The model under review builds one solid part; all positions refer to its coordinate system, in mm. Coordinates: 2 decimals unless noted, no trailing zeros. Write each loop counter-clockwise with the first axis right and the second up, starting at its lowest first coordinate (ties: lowest second). Pieces come first, ordered by that corner, then holes. Notation, with made-up numbers: (-9.5, -38.5) - (10.5, -38.5) arc R29 ccw to (10.5, -2.5) - close; hole circle Ø1 at (-27, 21). An arc over 180 degrees is marked (long way). Put each result on its own line as item: value.
Autodesk Inventor part; units mm, degrees
ref_plane "YZ Plane" through (0, 0, 0) normal (1, 0, 0) x (0, 1, 0)
ref_plane "XZ Plane" through (0, 0, 0) normal (0, 1, 0) x (-1, 0, 0)
ref_plane "XY Plane" through (0, 0, 0) normal (0, 0, 1) x (1, 0, 0)
sketch "Sketch3" plane through (0, 0, 0) normal (0, 1, 0) x (-1, 0, 0)
  line L0 (50, 50) -> (-50, 50)
  line L1 (-50, 50) -> (-50, -50)
  line L2 (-50, -50) -> (50, -50)
  line L3 (50, -50) -> (50, 50)
  line L4 (-50, -45) -> (50, -45) construction
  line L5 (-50, 45) -> (50, 45) construction
  line L6 (22.5, 50) -> (22.5, -50) construction
  line L7 (-22.5, 50) -> (-22.5, -50) construction
  circle A0 centre (-22.5, -45) radius 1.575
  circle A1 centre (-22.5, 45) radius 1.575
  circle A2 centre (22.5, 45) radius 1.575
  circle A3 centre (22.5, -45) radius 1.575
  point P0 (0, 0)
  dimension "d4" = 100
  dimension "d5" = 100
  dimension "d6" = 5
  dimension "d7" = 5
  dimension "d8" = 27.5
  dimension "d9" = 27.5
  dimension "d10" = 3.15
  dimension "d11" = 3.15
  dimension "d12" = 3.15
  dimension "d13" = 3.15
extrude "Extrusion1" add sketch "Sketch3" along normal blind 1
properties part number "CompCellScopeArray"
1. Consider section A-A on z = 45. State the section outline as (x, y) points (3 decimals).
Determined:
outline: (-50, 0) - (-24.075, 0) - (-24.075, 1) - (-50, 1) - close; (-20.925, 0) - (20.925, 0) - (20.925, 1) - (-20.925, 1) - close; (24.075, 0) - (50, 0) - (50, 1) - (24.075, 1) - close
2. To check wall thickness, follow probe 1 along Z at (x, y) = (-22.5, 0.5) (3 decimals). State the ranges of the line that lie inside material, in increasing order.
Determined:
probe 1: z = -50 to -46.575, -43.425 to 43.425, 46.575 to 50
3. The part is to be moulded in two halves that separate along X. For faces 1 (the cylindrical face through (23.661, 0.493, 43.936)), 2 (the flat face through (1, 0, 1)), say which applies: +X half, -X half, draft (parallel to the pull), parting line (faces both ways), or undercut.
Determined:
face 1: undercut
face 2: draft
4. Consider section B-B on x = -22.5. State the section outline as (y, z) points (3 decimals), plus the area to 3 significant figures.
Determined:
outline: (0, -50) - (1, -50) - (1, -46.575) - (0, -46.575) - close; (0, -43.425) - (1, -43.425) - (1, 43.425) - (0, 43.425) - close; (0, 46.575) - (1, 46.575) - (1, 50) - (0, 50) - close
area: 93.7 mm^2
5. For pin 1 Ø2.5 at (x, z) = (22.5, -45) entering from +Y, flat-tipped, find the tip position at first contact; note if it passes through.
Determined:
pin 1: passes through
